Autodesk Inventor part; units mm, degrees
ref_plane "YZ Plane" through (0, 0, 0) normal (1, 0, 0) x (0, 1, 0)
ref_plane "XZ Plane" through (0, 0, 0) normal (0, 1, 0) x (-1, 0, 0)
ref_plane "XY Plane" through (0, 0, 0) normal (0, 0, 1) x (1, 0, 0)
sketch "Sketch3" plane through (0, 0, 0) normal (0, 1, 0) x (-1, 0, 0)
  circle A0 centre (0, 0) radius 11
  circle A1 centre (0, 0) radius 17.5 construction
  circle A2 centre (0, 0) radius 40 construction
  circle A3 centre (0, 0) radius 54
  line L0 (-10, 38.7298) -> (-5, 16.7705)
  line L1 (10, 38.7298) -> (5, 16.7705)
  arc A4 (10, 38.7298) -> (-10, 38.7298) centre (0, 0) ccw
  arc A5 (5, 16.7705) -> (-5, 16.7705) centre (0, 0) ccw
  circle A6 centre (0, 0) radius 30 construction
  line L2 (7.7787, 28.974) -> (21.2029, 21.2235) construction
  line L3 (14.4908, 25.0988) -> (15, 25.9808) construction
  circle A7 centre (15, 25.9808) radius 2.5
  circle A8 centre (-15, 25.9808) radius 2.5
  circle A9 centre (-30, 0) radius 2.5
  circle A10 centre (-15, -25.9808) radius 2.5
  circle A11 centre (15, -25.9808) radius 2.5
  circle A12 centre (30, 0) radius 2.5
  arc A13 (-28.541, 28.0252) -> (-38.541, 10.7047) centre (0, 0) ccw
  line L4 (-28.541, 28.0252) -> (-12.0237, 12.7154)
  line L5 (-38.541, 10.7047) -> (-17.0237, 4.0551)
  arc A14 (-12.0237, 12.7154) -> (-17.0237, 4.0551) centre (0, 0) ccw
  arc A15 (-38.541, -10.7047) -> (-28.541, -28.0252) centre (0, 0) ccw
  line L6 (-38.541, -10.7047) -> (-17.0237, -4.0551)
  line L7 (-28.541, -28.0252) -> (-12.0237, -12.7154)
  arc A16 (-17.0237, -4.0551) -> (-12.0237, -12.7154) centre (0, 0) ccw
  arc A17 (-10, -38.7298) -> (10, -38.7298) centre (0, 0) ccw
  line L8 (-10, -38.7298) -> (-5, -16.7705)
  line L9 (10, -38.7298) -> (5, -16.7705)
  arc A18 (-5, -16.7705) -> (5, -16.7705) centre (0, 0) ccw
  arc A19 (28.541, -28.0252) -> (38.541, -10.7047) centre (0, 0) ccw
  line L10 (28.541, -28.0252) -> (12.0237, -12.7154)
  line L11 (38.541, -10.7047) -> (17.0237, -4.0551)
  arc A20 (12.0237, -12.7154) -> (17.0237, -4.0551) centre (0, 0) ccw
  arc A21 (38.541, 10.7047) -> (28.541, 28.0252) centre (0, 0) ccw
  line L12 (38.541, 10.7047) -> (17.0237, 4.0551)
  line L13 (28.541, 28.0252) -> (12.0237, 12.7154)
  arc A22 (17.0237, 4.0551) -> (12.0237, 12.7154) centre (0, 0) ccw
  point P0 (-21.2029, 21.2235)
  point P1 (-28.9815, -7.7505)
  point P2 (-7.7787, -28.974)
  point P3 (21.2029, -21.2235)
  point P4 (28.9815, 7.7505)
  dimension "d16" = 22
  dimension "d17" = 35
  dimension "d18" = 80
  dimension "d19" = 108
  dimension "d20" = 10
  dimension "d21" = 5
  dimension "d22" = 10
  dimension "d23" = 5
  dimension "d28" = 60
  dimension "d29" = 5
  dimension "d32" = 360
  dimension "d38" = 360
extrude "Extrusion4" add sketch "Sketch3" along normal blind 7
sketch "Sketch4" plane through (0, 7, 0) normal (0, 1, 0) x (1, 0, 0)
  circle A0 centre (0, 0) radius 47.5
  circle A1 centre (0, 0) radius 46.5
  dimension "d42" = 95
  dimension "d43" = 93
extrude "Extrusion5" add sketch "Sketch4" along normal blind 4
sketch "Sketch6" plane through (0, 11, 0) normal (0, 1, 0) x (1, 0, 0)
  circle A0 centre (0, 0) radius 46.5
  circle A1 centre (0, 0) radius 48
  dimension "d49" = 96
extrude "Extrusion7" add sketch "Sketch6" along normal blind 1
properties part number "Flexspline" material "ABS Plastic"
Work out the finished part from the listing and answer in its coordinate system (mm). A direction names the side the tool comes from. Give positions to 0.01 mm unless a question says otherwise; leave off trailing zeros. Order: outer loops, then holes, each group sorted by start corner. A loop starts at its lowest first (then second) coordinate and runs counter-clockwise, first axis right, second up.
1. For faces 1 (the flat face through (-25.11, 12, -39.34)), 2 (the cylindrical face through (-34.57, 3.45, 20.12)), 3 (the flat face through (-46.4, 11, -10.9)), determine the directions among +Z, -Z, +X, -X, +Y, -Y from which every point of the face is accessible in a straight line to the end or side of a thin tool.
Result sheet:
face 1: +Z, -Z, +X, -X, +Y
face 2: +Y, -Y
face 3: none
2. Each of these flat-tipped pins is pushed along its axis until it touches: P1, Ø6.5, axis at x = -15, z = -25.98, coming from the +Y side; P2, Ø1.5, axis at x = -19, y = 4.5, coming from the -Z side; P3, Ø4.5, axis at x = 15, z = -25.98, coming from the +Y side; P4, Ø1, axis at y = 8, z = -2, coming from the -X side. Where does it stop, or does it pass through?
Result sheet:
P1: stops at y = 7
P2: stops at z = -50.82
P3: passes through
P4: stops at x = -47.48
3. Section D-D, the plane z = 30 is taken. Determine the outline of the cut face in (x, y).
Result sheet:
outline: (-44.9, 0) - (-8.01, 0) - (-8.01, 7) - (-35.53, 7) - (-35.53, 12) - (-37.47, 12) - (-37.47, 11) - (-36.83, 11) - (-36.83, 7) - (-44.9, 7) - close; (8.01, 0) - (44.9, 0) - (44.9, 7) - (36.83, 7) - (36.83, 11) - (37.47, 11) - (37.47, 12) - (35.53, 12) - (35.53, 7) - (8.01, 7) - close
4. Section C-C, the plane x = 30 is taken. Determine the outline of the cut face in (y, z), and give its area (3 significant figures).
Result sheet:
outline: (0, -44.9) - (7, -44.9) - (7, -36.83) - (11, -36.83) - (11, -37.47) - (12, -37.47) - (12, -35.53) - (7, -35.53) - (7, -26.46) - (0, -26.46) - close; (0, -8.07) - (7, -8.07) - (7, -2.5) - (0, -2.5) - close; (0, 2.5) - (7, 2.5) - (7, 8.07) - (0, 8.07) - close; (0, 26.46) - (7, 26.46) - (7, 35.53) - (12, 35.53) - (12, 37.47) - (11, 37.47) - (11, 36.83) - (7, 36.83) - (7, 44.9) - (0, 44.9) - close
area: 350 mm2
5. Straight lines are drawn through the part: L1, parallel to Z at x = 0, y = 8.15; L2, parallel to Z at x = -24.5, y = 2.75; L3, parallel to X at y = 5, z = 1. For each, find the intervals that lie inside material, in ascending order.
Result sheet:
L1: z = -47.5 to -46.5, 46.5 to 47.5
L2: z = -48.12 to -24.28, -6.37 to 6.37, 24.28 to 48.12
L3: x = -53.99 to -32.29, -27.71 to -10.95, 10.95 to 27.71, 32.29 to 53.99
6. The mould has two halves that part along X. Classify faces 4 (the flat face through (0, 7, -48)), 5 (the cylindrical face through (-34.7, 3.5, -19.9)), 6 (the cylindrical face through (11.706, 3.451, 52.716)), 7 (the flat face through (20.4, 3.45, -20.48)): released by +X, released by -X, zero draft, split by the parting line, or undercut.
Result sheet:
face 4: zero draft
face 5: undercut
face 6: split by the parting line
face 7: undercut
7. Section B-B, the plane x = 15 is taken. Give the number of separate pieces and of enclosed holes in the cut face, and give its area (3 significant figures).
Result sheet:
separate pieces: 5
enclosed holes: 0
area: 577 mm2
8. Section A-A, the plane z = 0 is taken. Determine the outline of the cut face in (x, y), and give its area (3 significant figures).
Result sheet:
outline: (-54, 0) - (-32.5, 0) - (-32.5, 7) - (-46.5, 7) - (-46.5, 12) - (-48, 12) - (-48, 11) - (-47.5, 11) - (-47.5, 7) - (-54, 7) - close; (-27.5, 0) - (-11, 0) - (-11, 7) - (-27.5, 7) - close; (11, 0) - (27.5, 0) - (27.5, 7) - (11, 7) - close; (32.5, 0) - (54, 0) - (54, 7) - (47.5, 7) - (47.5, 11) - (48, 11) - (48, 12) - (46.5, 12) - (46.5, 7) - (32.5, 7) - close
area: 543 mm2
